Can you work these out from the model? Positions are in its coordinate system, mm. Face numbers are marked on the shaded views. A direction names the side the tool comes from. Round coordinates to 2 decimals unless told otherwise and drop trailing zeros. Loops run counter-clockwise (first coordinate to the right, second up) from the corner with the lowest first, then second, coordinate; pieces in that order, holes last.
(1) If I drill on line 1 along X through (y, z) = (8, 3.5); line 2 along Z through (x, y) = (-90.5, 62.5); line 3 along X through (y, z) = (-12, -62.5), over which ranges is the centre line in solid material (lowest first)?
(2) I want a section at D-D on x = 9.5. Write out the boundary of the cut face in (y, z), plus the area to 3 significant figures.
(3) I want a section at A-A on y = 33.5. Write out the boundary of the cut face in (x, z), plus the area to 3 significant figures.
(4) I want a section at B-B on z = 4. Give the number of separate pieces and of enclosed holes in the cut face, plus the area to 3 significant figures.
(5) Which directions (+Z, -Z, +X, -X, +Y, -Y) give clear straight access to the entire face, cutting with the end or side of a thin tool? Please do the marked faces 1 and 2.
(6) Will these pins go through, and if not, where does the flat tip stop? pin 1 Ø8.5 at (x, y) = (-83.54, -15.2) entering from -Z; pin 2 Ø12 at (x, z) = (-164, 7) entering from -Y; pin 3 Ø8 at (y, z) = (-6, -39.5) entering from +X.
(7) I want a section at C-C on y = 59.5. Write out the boundary of the cut face in (x, z), plus the area to 3 significant figures.
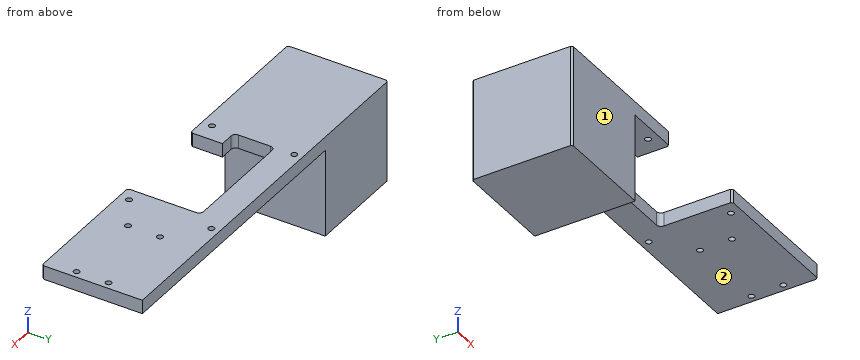
from build123d import *

# Parameters (mm, degrees)
F0_W      = 430
F0_H      = 110
F1_DEPTH  = 15
F2_W      = 130
F2_H      = 45
F3_DEPTH  = 25
F4_W      = 110
F4_H      = 45.9024896845
F5_DEPTH  = 25
F6_R      = 5
F7_SIZE   = 2
F9_DEPTH  = 96
F11_R     = 3.25
F12_DEPTH = 25
F13_R     = 3.25
F14_DEPTH = 25


with BuildPart() as f1:
    # F0 (on Top) → F1 (new body)
    with BuildSketch(Plane.XY):
        with Locations((-163.5564976931, 28.7499989569)):
            Rectangle(F0_W, F0_H)
    extrude(amount=F1_DEPTH)

    # F2 (on Top) → F3 (cut)
    with BuildSketch(Plane.XY):
        with Locations((-163.5564976931, 31.2499989569)):
            Rectangle(F2_W, F2_H)
    extrude(amount=F3_DEPTH, mode=Mode.SUBTRACT)

    # F4 (on Top) → F5 (cut)
    with BuildSketch(Plane.XY):
        with Locations((-153.5564976931, -10.6971156783)):
            Rectangle(F4_W, F4_H)
    extrude(amount=F5_DEPTH, mode=Mode.SUBTRACT)

    # F6
    f6_edges = [f1.edges().sort_by_distance(p)[0] for p in [
        (-228.556498, 53.749999, 7.5),
        (-98.556498, 53.749999, 7.5),
        (-228.556498, 8.749999, 7.5),
    ]]
    fillet(f6_edges, radius=F6_R)

    # F7
    f7_edges = [f1.edges().sort_by_distance(p)[0] for p in [
        (-208.556498, -26.250001, 7.5),
        (-98.556498, -26.250001, 7.5),
        (-378.556498, -26.250001, 7.5),
        (-378.556498, 83.749999, 7.5),
        (51.443502, -26.250001, 7.5),
    ]]
    chamfer(f7_edges, length=F7_SIZE)

    # F8 (on face) → F9 (join)
    with BuildSketch(Plane(origin=(0, 0, 0), x_dir=(1, 0, 0), z_dir=(0, 0, -1))):
        Polygon((-268.5564976931, 26.2500010431), (-376.5564976931, 26.2500010431), (-378.5564976931, 24.2500010431), (-378.5564976931, -81.7499989569), (-376.5564976931, -83.7499989569), (-268.5564976931, -83.7499989569), align=None)
    extrude(amount=F9_DEPTH)

    # F11 (on Top) → F12 (cut)
    with BuildSketch(Plane.XY):
        with Locations((-228.5088598728, -15.1645448059)):
            Circle(F11_R)
        with Locations((-228.553250432, 74.8012885451)):
            Circle(F11_R)
        with Locations((-83.5528895259, 74.8062729836)):
            Circle(F11_R)
        with Locations((-83.5413336754, -15.1974624023)):
            Circle(F11_R)
    extrude(amount=F12_DEPTH, mode=Mode.SUBTRACT)

    # F13 (on Top) → F14 (cut)
    with BuildSketch(Plane.XY):
        with Locations((-46.5564976931, 6.8009085655)):
            Circle(F13_R)
        with Locations((-46.5564976931, 41.8009085655)):
            Circle(F13_R)
        with Locations((43.4435023069, 6.8009085655)):
            Circle(F13_R)
        with Locations((43.4435023069, 41.8009085655)):
            Circle(F13_R)
    extrude(amount=F14_DEPTH, mode=Mode.SUBTRACT)


solid = f1.part
Filled sheet:
1. line 1: x = -378.56 to -208.56, -98.56 to -49.58, -43.54 to 40.42, 46.46 to 51.44
1. line 2: z = 0 to 15
1. line 3: x = -378.56 to -268.56
2. outline: (-26.25, 0) - (83.75, 0) - (83.75, 15) - (-26.25, 15) - close
2. area: 1,650 mm2
3. outline: (-378.56, -96) - (-268.56, -96) - (-268.56, 0) - (-228.56, 0) - (-228.56, 15) - (-378.56, 15) - close; (-98.56, 0) - (51.44, 0) - (51.44, 15) - (-98.56, 15) - close
3. area: 15,100 mm2
4. separate pieces: 1
4. enclosed holes: 8
4. area: 37,300 mm2
5. face 1: +Z, -Z, +X, -X, -Y
5. face 2: -Z, +X, +Y, -Y
6. pin 1: stops at z = 0
6. pin 2: stops at y = 53.75
6. pin 3: stops at x = -268.56
7. outline: (-378.56, -96) - (-268.56, -96) - (-268.56, 0) - (51.44, 0) - (51.44, 15) - (-378.56, 15) - close
7. area: 17,000 mm2
